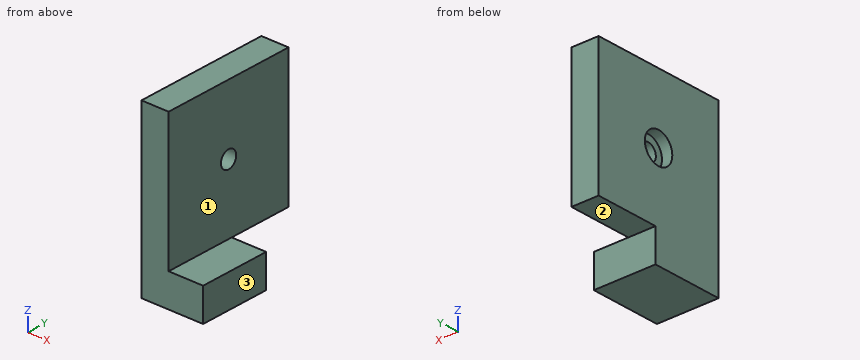
```python
from build123d import *

# Parameters (mm, degrees)
F0_W           = 13.1409592241
F0_H           = 6
F1_DEPTH       = 5
F3_D           = 3.175
F3_CBORE_D     = 5.715
F3_CBORE_DEPTH = 1.905
F4_W           = 13.1409592241
F4_H           = 6
F5_DEPTH       = 6.35


with BuildPart() as f1:
    # F0 (on Right) → F1 (new body)
    with BuildSketch(Plane.YZ):
        with Locations((-33.4253355518, -3)):
            Rectangle(F0_W, F0_H)
        Polygon((-14.9958151639, 25), (-39.9958151639, 25), (-39.9958151639, 0), (-26.8548559397, 0), (-14.9958151639, 0), align=None)
    extrude(amount=F1_DEPTH)

    # F3 (through all)
    with Locations(Plane(origin=(0, 0, 0), x_dir=(0, -1, 0), z_dir=(-1, 0, 0))):
        with Locations((27.4958151639, 12.5)):
            CounterBoreHole(F3_D / 2, F3_CBORE_D / 2, F3_CBORE_DEPTH)

    # F4 (on face) → F5 (join)
    with BuildSketch(Plane.YZ.offset(5)):
        with Locations((-33.4253355518, -3)):
            Rectangle(F4_W, F4_H)
    extrude(amount=F5_DEPTH)


solid = f1.part
```
Input: part model. Units: mm. Frame: model coordinates. Face numbers are marked on the shaded views. A direction names the side the tool comes from. Coordinates: 2 decimals unless noted, no trailing zeros. Order: outer loops, then holes, each group sorted by start corner. A loop starts at its lowest first (then second) coordinate and runs counter-clockwise, first axis right, second up. Notation, with made-up numbers: (-11, 38) - (25, 38) arc R27 cw to (25, 76) - close; hole circle Ø4 at (71.25, 3.5). An arc over 180 degrees is marked (long way). Return JSON: item names as keys, results as strings.
Q1. Cut plane D-D (x = 6.5). Return loops of the section in (y, z).
The answers:
{"outline": "(-40, -6) - (-26.85, -6) - (-26.85, 0) - (-40, 0) - close"}
Q2. Cut plane B-B (x = 1). Return loops of the section in (y, z) (1 decimal), then the cut area to 3 significant figures.
The answers:
{"outline": "(-40, -6) - (-26.9, -6) - (-26.9, 0) - (-15, 0) - (-15, 25) - (-40, 25) - close; hole circle Ø5.7 at (-27.5, 12.5)", "area": "678 mm2"}
Q3. First-contact query: pin 1 (2 mm diameter, centred on y = -22.5, z = 13.5, fed in from +X); pin 2 (3 mm diameter, centred on x = 7.5, z = -1.5, fed in from +Y); pin 3 (3 mm diameter, centred on y = -27.5, z = 13, fed in from -X) (3 decimals). Flat tips, straight axial feed; report the tip coordinate or a pass-through.
The answers:
{"pin 1": "stops at x = 5", "pin 2": "stops at y = -26.85", "pin 3": "stops at x = 1.905"}
Q4. Access query for the marked faces 1, 2 and 3. Directions: +Z, -Z, +X, -X, +Y, -Y. A direction counts if a zero-diameter tool reaches every point of the face in a straight line with its end or side. Return the directions, or none.
The answers:
{"face 1": "+Z, +X, +Y, -Y", "face 2": "-Z, +X, -X, +Y", "face 3": "+Z, -Z, +X, +Y, -Y"}
Q5. Ray query, probe 1 along Z at (x, y) = (10, -33); probe 2 along Y at (x, z) = (5, -3.5); probe 3 along Z at (x, y) = (2, -23). Return the intervals inside material, ascending.
The answers:
{"probe 1": "z = -6 to 0", "probe 2": "y = -40 to -26.85", "probe 3": "z = 0 to 25"}
Q6. Cut plane C-C (z = 20). Return loops of the section in (x, y), then the cut area to 3 significant figures.
The answers:
{"outline": "(0, -40) - (5, -40) - (5, -15) - (0, -15) - close", "area": "125 mm2"}
Q7. Cut plane A-A (z = 12.5). Return loops of the section in (x, y) (3 decimals).
The answers:
{"outline": "(0, -39.996) - (5, -39.996) - (5, -29.083) - (1.905, -29.083) - (1.905, -30.353) - (0, -30.353) - close; (0, -24.638) - (1.905, -24.638) - (1.905, -25.908) - (5, -25.908) - (5, -14.996) - (0, -14.996) - close"}
